The listing builds one solid part. Answer for the finished solid, in the listing's coordinates (mm). A direction names the side the tool comes from. Coordinates: 2 decimals unless noted, no trailing zeros. Loops run counter-clockwise (first coordinate to the right, second up) from the corner with the lowest first, then second, coordinate; pieces in that order, holes last. Notation, with made-up numbers: (41.25, 38.5) - (45.25, 38.5) arc R31 ccw to (45.25, 75.5) - close; hole circle Ø5 at (-19, 78). An arc over 180 degrees is marked (long way). One line per question, with ' | ' between items.
from build123d import *

# Parameters (mm, degrees)
BOSS_EXTRUDE1_DEPTH = 12.7
SKETCH2_R           = 2.286
CUT_EXTRUDE1_DEPTH  = 32.908355097
SKETCH3_R           = 4.445
CUT_EXTRUDE2_DEPTH  = 2.54
SKETCH4_R           = 1.905
CUT_EXTRUDE3_DEPTH  = 12.7
SKETCH5_R           = 1.905
CUT_EXTRUDE4_DEPTH  = 12.7
FILLET1_R           = 1.5875
FILLET2_R           = 0.79375


with BuildPart() as part:
    # Sketch1 → Boss-Extrude1 (new body)
    with BuildSketch(Plane(origin=(0, 0, 0), x_dir=(1, 0, 0), z_dir=(0, 1, 0))):
        Polygon((-19.05, 0), (19.05, 0), (19.05, -11.1125), (6.35, -22.225), (-19.05, -22.225), align=None)
    extrude(amount=BOSS_EXTRUDE1_DEPTH)

    # Sketch2 → Cut-Extrude1 (cut, through all)
    with BuildSketch(Plane(origin=(0, 12.7, 0), x_dir=(1, 0, 0), z_dir=(0, 1, 0))):
        with Locations(Location((0, -4.7625, 0), (0, 0, 270))):
            Circle(SKETCH2_R)
        with Locations(Location((-12.7, -17.4625, 0), (0, 0, 270))):
            Circle(SKETCH2_R)
    extrude(amount=-CUT_EXTRUDE1_DEPTH, mode=Mode.SUBTRACT)

    # Sketch3 → Cut-Extrude2 (cut)
    with BuildSketch(Plane(origin=(0, 12.7, 0), x_dir=(1, 0, 0), z_dir=(0, 1, 0))):
        with Locations(Location((0, -4.7625, 0), (0, 0, 270))):
            Circle(SKETCH3_R)
        with Locations(Location((-12.7, -17.4625, 0), (0, 0, 270))):
            Circle(SKETCH3_R)
    extrude(amount=-CUT_EXTRUDE2_DEPTH, mode=Mode.SUBTRACT)

    # Sketch4 → Cut-Extrude3 (cut)
    with BuildSketch(Plane(origin=(0, 0, 0), x_dir=(-1, 0, 0), z_dir=(0, 0, -1))):
        with Locations((-12.7, 6.35)):
            Circle(SKETCH4_R)
        with Locations((12.7, 6.35)):
            Circle(SKETCH4_R)
    extrude(amount=-CUT_EXTRUDE3_DEPTH, mode=Mode.SUBTRACT)

    # Sketch5 → Cut-Extrude4 (cut)
    with BuildSketch(Plane.XY.offset(22.225)):
        with Locations((0, 6.35)):
            Circle(SKETCH5_R)
    extrude(amount=-CUT_EXTRUDE4_DEPTH, mode=Mode.SUBTRACT)

    # Fillet1
    fillet1_edges = [part.edges().sort_by_distance(p)[0] for p in [
        (-19.05, 0, 11.1125),
        (0, 0, 0),
        (19.05, 0, 5.55625),
        (12.7, 0, 16.66875),
        (-6.35, 0, 22.225),
        (-19.05, 6.35, 22.225),
        (-19.05, 6.35, 0),
        (19.05, 6.35, 0),
        (19.05, 6.35, 11.1125),
        (6.35, 6.35, 22.225),
    ]]
    fillet(fillet1_edges, radius=FILLET1_R)

    # Fillet2
    # the kernel refuses this fillet: 0.79375 mm, written as the material it takes off along each edge
    with BuildSketch(Plane(origin=(0, 12.7, 4.7625), x_dir=(0, 0, 1), z_dir=(-1, 0, 0))) as fillet2_piece_1:
        with BuildLine():
            CenterArc((4.445 + FILLET2_R, -FILLET2_R), FILLET2_R, 90, 90)
            Line((4.445, -FILLET2_R), (4.445, 0))
            Line((4.445, 0), (4.445 + FILLET2_R, 0))
        make_face()
    revolve(axis=Axis((0, 12.7, 4.7625), (0, 1, 0)), mode=Mode.SUBTRACT)
    with BuildSketch(Plane(origin=(-12.7, 12.7, 17.4625), x_dir=(0, 0, 1), z_dir=(-1, 0, 0))) as fillet2_piece_2:
        with BuildLine():
            CenterArc((4.445 + FILLET2_R, -FILLET2_R), FILLET2_R, 90, 90)
            Line((4.445, -FILLET2_R), (4.445, 0))
            Line((4.445, 0), (4.445 + FILLET2_R, 0))
        make_face()
    revolve(axis=Axis((-12.7, 12.7, 17.4625), (0, 1, 0)), mode=Mode.SUBTRACT)
    with BuildSketch(Plane(origin=(-17.4625, 12.7, 0), x_dir=(0, -1, 0), z_dir=(1, 0, 0))) as fillet2_piece_3:
        with BuildLine():
            CenterArc((FILLET2_R, -FILLET2_R), FILLET2_R, 90, 90)
            Line((0, -FILLET2_R), (0, 0))
            Line((0, 0), (FILLET2_R, 0))
        make_face()
    extrude(amount=34.925, mode=Mode.SUBTRACT)
    with BuildSketch(Plane(origin=(19.05, 12.7, 1.5875), x_dir=(-1, 0, 0), z_dir=(0, 0, 1))) as fillet2_piece_4:
        with BuildLine():
            CenterArc((FILLET2_R, FILLET2_R), FILLET2_R, 180, 90)
            Line((0, FILLET2_R), (0, 0))
            Line((0, 0), (FILLET2_R, 0))
        make_face()
    extrude(amount=8.80464294, mode=Mode.SUBTRACT)
    with BuildSketch(Plane(origin=(5.753520503, 12.7, 22.225), x_dir=(0, 0, -1), z_dir=(-1, 0, 0))) as fillet2_piece_5:
        with BuildLine():
            CenterArc((FILLET2_R, FILLET2_R), FILLET2_R, 180, 90)
            Line((0, FILLET2_R), (0, 0))
            Line((0, 0), (FILLET2_R, 0))
        make_face()
    extrude(amount=23.216020503, mode=Mode.SUBTRACT)
    with BuildSketch(Plane(origin=(18.507876065, 12.7, 11.586858443), x_dir=(-0.6585046078685184, 0, -0.7525766947068776), z_dir=(-0.7525766947068777, 0, 0.6585046078685184))) as fillet2_piece_6:
        with BuildLine():
            CenterArc((FILLET2_R, FILLET2_R), FILLET2_R, 180, 90)
            Line((0, FILLET2_R), (0, 0))
            Line((0, 0), (FILLET2_R, 0))
        make_face()
    extrude(amount=15.558519921, mode=Mode.SUBTRACT)
    with BuildSketch(Plane(origin=(-19.05, 12.7, 20.6375), x_dir=(1, 0, 0), z_dir=(0, 0, -1))) as fillet2_piece_7:
        with BuildLine():
            CenterArc((FILLET2_R, FILLET2_R), FILLET2_R, 180, 90)
            Line((0, FILLET2_R), (0, 0))
            Line((0, 0), (FILLET2_R, 0))
        make_face()
    extrude(amount=19.05, mode=Mode.SUBTRACT)
    with BuildSketch(Plane(origin=(-17.4625, 12.7, 20.6375), x_dir=(-1, 0, 0), z_dir=(0, 0, -1))) as fillet2_piece_8:
        with BuildLine():
            CenterArc((1.5875 - FILLET2_R, -FILLET2_R), FILLET2_R, 0, 90)
            Line((1.5875, -FILLET2_R), (1.5875, 0))
            Line((1.5875, 0), (1.5875 - FILLET2_R, 0))
        make_face()
    revolve(axis=Axis((-17.4625, 12.7, 20.6375), (0, 1, 0)), revolution_arc=90, mode=Mode.SUBTRACT)
    with BuildSketch(Plane(origin=(-17.4625, 12.7, 1.5875), x_dir=(0, 0, -1), z_dir=(1, 0, 0))) as fillet2_piece_9:
        with BuildLine():
            CenterArc((1.5875 - FILLET2_R, -FILLET2_R), FILLET2_R, 0, 90)
            Line((1.5875, -FILLET2_R), (1.5875, 0))
            Line((1.5875, 0), (1.5875 - FILLET2_R, 0))
        make_face()
    revolve(axis=Axis((-17.4625, 12.7, 1.5875), (0, 1, 0)), revolution_arc=90, mode=Mode.SUBTRACT)
    with BuildSketch(Plane(origin=(5.753520503, 12.7, 20.6375), x_dir=(0, 0, 1), z_dir=(-1, 0, 0))) as fillet2_piece_10:
        with BuildLine():
            CenterArc((1.5875 - FILLET2_R, -FILLET2_R), FILLET2_R, 0, 90)
            Line((1.5875, -FILLET2_R), (1.5875, 0))
            Line((1.5875, 0), (1.5875 - FILLET2_R, 0))
        make_face()
    revolve(axis=Axis((5.753520503, 12.7, 20.6375), (0, 1, 0)), revolution_arc=41.185925166, mode=Mode.SUBTRACT)
    with BuildSketch(Plane(origin=(17.4625, 12.7, 10.39214294), x_dir=(1, 0, 0), z_dir=(0, 0, -1))) as fillet2_piece_11:
        with BuildLine():
            CenterArc((1.5875 - FILLET2_R, FILLET2_R), FILLET2_R, 270, 90)
            Line((1.5875, FILLET2_R), (1.5875, 0))
            Line((1.5875, 0), (1.5875 - FILLET2_R, 0))
        make_face()
    revolve(axis=Axis((17.4625, 12.7, 10.39214294), (0, -1, 0)), revolution_arc=48.814074834, mode=Mode.SUBTRACT)
    with BuildSketch(Plane(origin=(17.4625, 12.7, 1.5875), x_dir=(0, 0, -1), z_dir=(-1, 0, 0))) as fillet2_piece_12:
        with BuildLine():
            CenterArc((1.5875 - FILLET2_R, FILLET2_R), FILLET2_R, 270, 90)
            Line((1.5875, FILLET2_R), (1.5875, 0))
            Line((1.5875, 0), (1.5875 - FILLET2_R, 0))
        make_face()
    revolve(axis=Axis((17.4625, 12.7, 1.5875), (0, -1, 0)), revolution_arc=90, mode=Mode.SUBTRACT)


solid = part.part
Item 1: The mould has two halves that part along X. Classify faces 4 (the face through (0, 0, 11)), 5 (the face through (18.57, 0.45, 6.05)), 6 (the face through (-12, 10.16, 15)): pulls with the +X half, pulls with the -X half, needs draft (parallel to the pull), parting line crosses it, or undercut.
Taken from the geometry:
face 4: needs draft | face 5: pulls with the +X half | face 6: undercut
Item 2: Each of these flat-tipped pins is pushed along its axis until it touches: pin 1 Ø2.5 at (x, y) = (12.7, 6.35) entering from -Z; pin 2 Ø3.5 at (x, y) = (0, 6.35) entering from +Z (3 decimals); pin 3 Ø1 at (x, z) = (-11, 15) entering from +Y. Where does it stop, or does it pass through?
Taken from the geometry:
pin 1: stops at z = 12.7 | pin 2: stops at z = 9.525 | pin 3: stops at y = 10.16
Item 3: Which of the six approach directions +Z, -Z, +X, -X, +Y, -Y give full straight-line access (tool end or side, diameter ignored) to faces 1 (the face through (0, 6, 9.525)), 2 (the face through (-13, 6, 12.7)), 3 (the face through (-8.95, 11.05, 19.85))?
Taken from the geometry:
face 1: +Z | face 2: -Z | face 3: +Y
Item 4: Find the intervals of material crossed by line 1 (X direction, y = 7.5, z = 2); line 2 (X direction, y = 10.5, z = 5); line 3 (X direction, y = 6.75, z = 19.5), in increasing order. Write a range as [from, to].
Taken from the geometry:
line 1: x = [-19.05, -14.22], [-11.18, 11.18], [14.22, 19.05] | line 2: x = [-19.05, -4.44], [4.44, 19.05] | line 3: x = [-19.05, -13.74], [-11.66, -1.86], [1.86, 9.46]
Item 5: Find section B-B, the plane x = -12.7. Write down the section's boundary in (y, z) (1 decimal), plus the area to 3 significant figures.
Taken from the geometry:
outline: (0, 1.6) arc R1.6 ccw to (1.6, 0) - (4.4, 0) - (4.4, 12.7) - (8.3, 12.7) - (8.3, 0) - (11.9, 0) arc R0.8 ccw to (12.7, 0.8) - (12.7, 12.2) arc R0.8 ccw to (11.9, 13) - (10.2, 13) - (10.2, 15.2) - (0, 15.2) - close; (0, 19.7) - (10.2, 19.7) - (10.2, 21.9) - (11.9, 21.9) arc R0.8 ccw to (12.4, 22.1) arc R0.8 ccw to (11.9, 22.2) - (1.6, 22.2) arc R1.6 ccw to (0, 20.6) - close | area: 163 mm2
Item 6: Find section A-A, the plane y = 6.35. State how many separate pieces and enclosed holes the cut face has, plus the area to 3 significant figures.
Taken from the geometry:
separate pieces: 1 | enclosed holes: 2 | area: 596 mm2
